Geometry: final body of the model. Coordinates: model frame, mm. A direction names the side the tool comes from. Give positions to 0.01 mm unless a question says otherwise; leave off trailing zeros. Write each loop counter-clockwise with the first axis right and the second up, starting at its lowest first coordinate (ties: lowest second). Pieces come first, ordered by that corner, then holes. Notation, with made-up numbers: (-8.5, -31.5) -> (22.5, -31.5) arc R13 ccw to (22.5, -19.5) -> close; hole circle Ø3 at (86.5, 58.5). An arc over 180 degrees is marked (long way). Answer as a JSON object with one key per item and string values. Group by question number.
(1) Material intervals for probe 1 along Y at (x, z) = (-9.5, 0.5); probe 2 along X at (y, z) = (-4.5, -1.5); probe 3 along Z at (x, y) = (-5, 2.75), sorted ascending.
(2) Section query B-B on z = -3. Output: boundary loops of the cut face in (x, y), plus the area to 3 significant figures.
(3) Set-up query: faces 1 (the face through (6, 3, 15.5)), 2 (the face through (-0.08, 5.43, -17.4)). Return all of +Z, -Z, +X, -X, +Y, -Y with unobstructed straight access to the full face (end or side cutting, diameter ignored); none if empty.
(4) Contact query for flat-ended pins moving along their axis: pin 1 Ø5 at (y, z) = (-13, 5) entering from +X; pin 2 Ø8 at (x, y) = (12, -3.5) entering from -Z; pin 3 Ø0.5 at (x, y) = (-15.5, 1.5) entering from +Z. Output: stop coordinate, or through.
(5) Section query D-D on z = 8. Output: boundary loops of the cut face in (x, y).
(6) Section query A-A on y = -2.25. Output: boundary loops of the cut face in (x, z), plus the area to 3 significant figures.
(7) Section query C-C on x = 3. Output: boundary loops of the cut face in (y, z).
Autodesk Inventor part; units mm, degrees
ref_plane "YZ Plane" through (0, 0, 0) normal (1, 0, 0) x (0, 1, 0)
ref_plane "XZ Plane" through (0, 0, 0) normal (0, 1, 0) x (-1, 0, 0)
ref_plane "XY Plane" through (0, 0, 0) normal (0, 0, 1) x (1, 0, 0)
sketch "Sketch1" plane through (0, 0, 0) normal (0, 1, 0) x (-1, 0, 0)
  circle A0 centre (0.1717, 0) radius 4.85
  line L0 (15, 15) -> (-15, 15)
  line L1 (-15, 15) -> (-15, -15)
  line L2 (-15, -15) -> (15, -15)
  line L3 (15, -15) -> (15, 15)
  line L4 (0, 15) -> (6, 15)
  line L5 (6, 15) -> (6, 18)
  line L6 (6, 18) -> (0, 18)
  line L7 (0, 18) -> (-6, 18)
  line L8 (-6, 18) -> (-6, 15)
  line L9 (-6, 15) -> (0, 15)
  line L10 (6, -15) -> (-6, -15)
  line L11 (-6, -15) -> (-6, -18)
  line L12 (-6, -18) -> (6, -18)
  line L13 (6, -18) -> (6, -15)
  line L14 (15, 6) -> (18, 6)
  line L15 (18, 6) -> (18, -6)
  line L16 (18, -6) -> (15, -6)
  line L17 (15, -6) -> (15, 6)
  line L18 (-15, -6) -> (-18, -6)
  line L19 (-18, -6) -> (-18, 6)
  line L20 (-18, 6) -> (-15, 6)
  line L21 (-15, 6) -> (-15, -6)
  arc A1 (15, 6) -> (6, 15) centre (6.5, 6.5) ccw
  arc A2 (6, -15) -> (15, -6) centre (4, -4) ccw
  arc A3 (-15, -6) -> (-6, -15) centre (-7, -7) ccw
  arc A4 (-6.3124, 15) -> (-15, 6) centre (-3.6523, 3.7392) ccw
  point P0 (0, 0)
  dimension "d0" = 9.7
extrude "Extrusion1" add sketch "Sketch1" along normal blind 6 contours L0 L8 L7 L6 L5 | L14 L15 L16 L3 | L1 L18 L19 L20 | L13 L12 L11 L2
extrude "Extrusion2" cut sketch "Sketch1" along normal blind 3 contours L0 A1 L3 A2 L2 A3 L1 A4 | A1 L0 | A1 L3 | L1 A3 | A3 L2
extrude "Extrusion3" add sketch "Sketch1" along normal blind 2 contours A0 | L0 A1 L3 A2 L2 A3 L1 A4 | A1 L0 | A1 L3 | L1 A3 | A3 L2
fillet "Fillet1" radius 2 12 edges at (18, 3, -6) (6, 3, -18) (-6, 3, -18) (-18, 3, -6) (-18, 3, 6) (-6, 3, 18) (6, 3, 18) (18, 3, 6) (0, 6, 18) (-18, 6, 0) (0, 6, -18) (18, 6, 0)
extrude "Extrusion4" add sketch "Sketch1" against normal blind 20 contours A0
properties part number "spider_support"
Answer list:
{
 "1": {"probe 1": "0 to 2", "probe 2": "-4.78 to 4.44", "probe 3": "-17.73 to -15, 15 to 17.73"},
 "2": {"outline": "(-18, 0) -> (-3.98, 0) -> (-3.98, -20) -> (3.64, -20) -> (3.64, 0) -> (18, 0) -> (18, 4) arc R2 ccw to (16, 6) -> (15, 6) -> (15, 2) -> (-15, 2) -> (-15, 6) -> (-16, 6) arc R2 ccw to (-18, 4) -> close", "area": "247 mm2"},
 "3": {"face 1": "+Z, +X, +Y, -Y", "face 2": "-Z, +X, -X, +Y"},
 "4": {"pin 1": "x = 3.98", "pin 2": "z = -14.46", "pin 3": "z = 6"},
 "5": {"outline": "(-14.88, 0) -> (14.41, 0) -> (14.41, 2) -> (-14.88, 2) -> close"},
 "6": {"outline": "circle Ø9.7 at (-0.17, 0)", "area": "73.9 mm2"},
 "7": {"outline": "(-20, -3.67) -> (0, -3.67) -> (0, -18) -> (4, -18) arc R2 ccw to (6, -16) -> (6, -15) -> (2, -15) -> (2, 15) -> (6, 15) -> (6, 16) arc R2 ccw to (4, 18) -> (0, 18) -> (0, 3.67) -> (-20, 3.67) -> close"}
}
